from build123d import *

# Parameters (mm, degrees)
SKETCH1_R               = 17.5
BOSS_EXTRUDE1_DEPTH     = 12
SHELL4_T                = -2
CUT_EXTRUDE1_DEPTH      = 28.504545079
CUT_EXTRUDE1_DEPTH_BACK = 28.504545079
SKETCH3_R               = 2.5
CUT_EXTRUDE2_DEPTH      = 28.504545079
CUT_EXTRUDE2_DEPTH_BACK = 28.504545079
SKETCH4_W               = 20
SKETCH4_H               = 24.94066955
BOSS_EXTRUDE2_DEPTH     = 12
FILLET1_R               = 2
FILLET2_R               = 2
FILLET5_R               = 1


with BuildPart() as part:
    # Sketch1 → Boss-Extrude1 (new body)
    with BuildSketch(Plane.XY):
        Circle(SKETCH1_R)
    extrude(amount=BOSS_EXTRUDE1_DEPTH)

    # Shell4
    shell4_openings = [part.faces().sort_by_distance(p)[0] for p in [
        (0, 0, 12),
    ]]
    offset(amount=SHELL4_T, openings=shell4_openings, kind=Kind.INTERSECTION)

    # Sketch3 → Cut-Extrude1 (cut, two sides: drawn at the far end of the back side and taken through both)
    with BuildSketch(Plane.XY.offset(-CUT_EXTRUDE1_DEPTH_BACK)):
        Circle(SKETCH3_R)
    extrude(amount=CUT_EXTRUDE1_DEPTH + CUT_EXTRUDE1_DEPTH_BACK, mode=Mode.SUBTRACT)

    # Sketch4 → Cut-Extrude2 (cut, two sides: drawn at the far end of the back side and taken through both)
    with BuildSketch(Plane(origin=(0, 0, 0), x_dir=(1, 0, 0), z_dir=(0, 1, 0)).offset(-CUT_EXTRUDE2_DEPTH_BACK)):
        with Locations((0, -14.470334775)):
            Rectangle(SKETCH4_W, SKETCH4_H)
    extrude(amount=CUT_EXTRUDE2_DEPTH + CUT_EXTRUDE2_DEPTH_BACK, mode=Mode.SUBTRACT)

    # Sketch7 → Boss-Extrude2 (add)
    with BuildSketch(Plane.XY.offset(12)):
        Polygon((-10, -14.361406616), (-10, -23.35781655), (-12, -23.35781655), (-13.169286174, -11.524751697), align=None)
        Polygon((10, -14.361406616), (10, -23.35781655), (12, -23.35781655), (13.169286174, -11.524751697), align=None)
    extrude(amount=-BOSS_EXTRUDE2_DEPTH)

    # Fillet1
    fillet1_edges = [part.edges().sort_by_distance(p)[0] for p in [
        (-10, -11.842719282, 7),
        (10, -11.842719282, 7),
    ]]
    fillet(fillet1_edges, radius=FILLET1_R)

    # Fillet2
    fillet2_edges = [part.edges().sort_by_distance(p)[0] for p in [
        (-13.169286174, -11.524751697, 6),
        (13.169286174, -11.524751697, 6),
    ]]
    fillet(fillet2_edges, radius=FILLET2_R)

    # Fillet5
    fillet5_edges = [part.edges().sort_by_distance(p)[0] for p in [
        (-10, -23.35781655, 6),
        (-12, -23.35781655, 6),
        (12, -23.35781655, 6),
        (10, -23.35781655, 6),
    ]]
    fillet(fillet5_edges, radius=FILLET5_R)


solid = part.part
Geometry: final body of the model. Coordinates: model frame, mm. A direction names the side the tool comes from. Coordinates: 2 decimals unless noted, no trailing zeros. Order: outer loops, then holes, each group sorted by start corner. A loop starts at its lowest first (then second) coordinate and runs counter-clockwise, first axis right, second up.
(1) Section query A-A (x = 0). Return the cut outline in (y, z).
(2) Access query for faces 1 (the face through (15.5, 0.2, 6.9)), 2 (the face through (10.29, -23.06, 5.92)), 3 (the face through (11.773, -23.092, 5.916)). Directions: +Z, -Z, +X, -X, +Y, -Y. A direction counts if a zero-diameter tool reaches every point of the face in a straight line with its end or side. Return the directions, or none.
(3) Section query B-B (z = 5.75). Return the cut outline in (x, y).
(4) Section query D-D (y = 5.5). Return the cut outline in (x, z).
(5) Section query C-C (y = 0). Return the cut outline in (x, z).
(6) Draft query along Y for faces 4 (the face through (-10, 13, 7)), 5 (the face through (10.159, -11.955, 6.93)), 6 (the face through (-10.3, -23.07, 5.92)). Return one class per face: pulls with the +Y half, pulls with the -Y half, needs draft (parallel to the pull), parting line crosses it, or undercut.
(7) First-contact query: pin 1 (3 mm diameter, centred on y = 13.5, z = 9, fed in from -X); pin 2 (4 mm diameter, centred on x = 8.5, z = 10, fed in from -Y); pin 3 (12 mm diameter, centred on x = -8.5, y = -3, fed in from +Z). Flat tips, straight axial feed; report the tip coordinate or a pass-through.
(8) Material intervals for probe 1 along X at (y, z) = (0.5, 3.25); probe 2 along Y at (x, z) = (0, 0.75), sorted ascending.
Solution:
1. outline: (-17.5, 0) - (-2.5, 0) - (-2.5, 2) - (-17.5, 2) - close; (2.5, 0) - (17.5, 0) - (17.5, 2) - (2.5, 2) - close
2. face 1: +Z
2. face 2: +Z, -Z, -Y
2. face 3: +Z, -Z, +X, -Y
3. outline: (-13.55, -11.07) arc R2 cw to (-13.11, -12.14) - (-12.09, -22.46) arc R1 ccw to (-11.09, -23.36) - (-11, -23.36) arc R1 ccw to (-10, -22.36) - (-10, -12.74) arc R2 ccw to (-10.63, -11.28) arc R15.5 cw to (-10, 11.84) - (-10, 14.36) arc R17.5 ccw to start; (10, -22.36) arc R1 ccw to (11, -23.36) - (11.09, -23.36) arc R1 ccw to (12.09, -22.46) - (13.11, -12.14) arc R2 cw to (13.55, -11.07) arc R17.5 ccw to (10, 14.36) - (10, 11.84) arc R15.5 cw to (10.63, -11.28) arc R2 ccw to (10, -12.74) - close
4. outline: (-16.61, 0) - (16.61, 0) - (16.61, 12) - (14.49, 12) - (14.49, 2) - (-14.49, 2) - (-14.49, 12) - (-16.61, 12) - close
5. outline: (-17.5, 0) - (-2.5, 0) - (-2.5, 2) - (-15.5, 2) - (-15.5, 12) - (-17.5, 12) - close; (2.5, 0) - (17.5, 0) - (17.5, 12) - (15.5, 12) - (15.5, 2) - (2.5, 2) - close
6. face 4: needs draft
6. face 5: undercut
6. face 6: pulls with the -Y half
7. pin 1: stops at x = -12.74
7. pin 2: stops at y = -23.22
7. pin 3: stops at z = 2
8. probe 1: x = -17.49 to -15.49, 15.49 to 17.49
8. probe 2: y = -17.5 to -2.5, 2.5 to 17.5
